Design review of the part built by this model. Coordinates are the model's own, in mm. Round coordinates to 2 decimals unless told otherwise and drop trailing zeros. Write each loop counter-clockwise with the first axis right and the second up, starting at its lowest first coordinate (ties: lowest second). Pieces come first, ordered by that corner, then holes. Notation, with made-up numbers: (59.25, 34.25) - (100.25, 34.25) arc R34 ccw to (100.25, 66.25) - close; hole circle Ø11 at (5.25, -29.75). An arc over 180 degrees is marked (long way). Use one line per item in the form item = value.
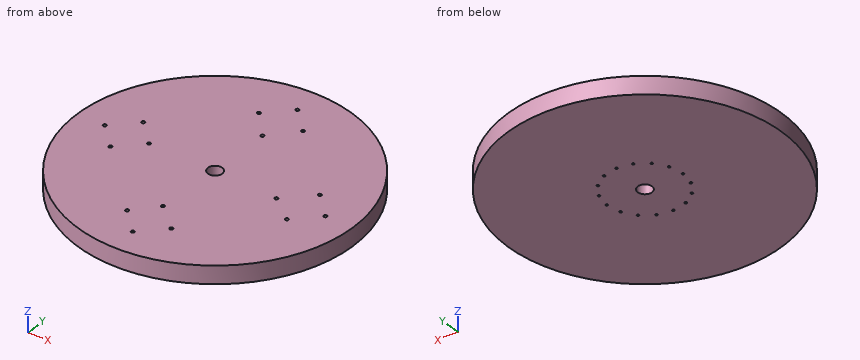
```python
from build123d import *

# Parameters (mm, degrees)
SKETCH_1_R               = 125
EXTRUDE_1_DEPTH          = 8.1
CUT_EXTRUDE_1_DEPTH      = 178.517435763
CUT_EXTRUDE_1_DEPTH_BACK = 178.517435763
SKETCH_3_R               = 6.52
SKETCH_2_R               = 1.03
CUT_EXTRUDE_4_DEPTH      = 10
SKETCH_7_R               = 1.5
CUT_EXTRUDE_5_DEPTH      = 10


with BuildPart() as part:
    # 草图1 → 凸台-拉伸1 (new, symmetric)
    with BuildSketch(Plane.XY):
        Circle(SKETCH_1_R)
    extrude(amount=EXTRUDE_1_DEPTH, both=True)

    # 草图3 → 切除-拉伸1 (cut, two sides: drawn at the far end of the back side and taken through both)
    with BuildSketch(Plane.XY.offset(8.1).offset(-CUT_EXTRUDE_1_DEPTH_BACK)):
        Circle(SKETCH_3_R)
    extrude(amount=CUT_EXTRUDE_1_DEPTH + CUT_EXTRUDE_1_DEPTH_BACK, mode=Mode.SUBTRACT)

    # 草图2 → 切除-拉伸4 (cut)
    with BuildSketch(Plane(origin=(0, 0, -8.1), x_dir=(-1, 0, 0), z_dir=(0, 0, -1))):
        with Locations((0, 34.5)):
            Circle(SKETCH_2_R)
        with Locations((13.202578417, 31.873843872)):
            Circle(SKETCH_2_R)
        with Locations((24.395183951, 24.395183951)):
            Circle(SKETCH_2_R)
        with Locations((31.873843872, 13.202578417)):
            Circle(SKETCH_2_R)
        with Locations((34.5, 0)):
            Circle(SKETCH_2_R)
        with Locations((31.873843872, -13.202578417)):
            Circle(SKETCH_2_R)
        with Locations((24.395183951, -24.395183951)):
            Circle(SKETCH_2_R)
        with Locations((13.202578417, -31.873843872)):
            Circle(SKETCH_2_R)
        with Locations((0, -34.5)):
            Circle(SKETCH_2_R)
        with Locations((-13.202578417, -31.873843872)):
            Circle(SKETCH_2_R)
        with Locations((-24.395183951, -24.395183951)):
            Circle(SKETCH_2_R)
        with Locations((-31.873843872, -13.202578417)):
            Circle(SKETCH_2_R)
        with Locations((-34.5, 0)):
            Circle(SKETCH_2_R)
        with Locations((-31.873843872, 13.202578417)):
            Circle(SKETCH_2_R)
        with Locations((-24.395183951, 24.395183951)):
            Circle(SKETCH_2_R)
        with Locations((-13.202578417, 31.873843872)):
            Circle(SKETCH_2_R)
    extrude(amount=-CUT_EXTRUDE_4_DEPTH, mode=Mode.SUBTRACT)

    # 草图7 → 切除-拉伸5 (cut)
    with BuildSketch(Plane.XY.offset(8.1)):
        with Locations((-100, 0)):
            Circle(SKETCH_7_R)
        with Locations((-80, 20)):
            Circle(SKETCH_7_R)
        with Locations((-60, 0)):
            Circle(SKETCH_7_R)
        with Locations((-80, -20)):
            Circle(SKETCH_7_R)
        with Locations((0, 57.5)):
            Circle(SKETCH_7_R)
        with Locations((57.5, -2.5)):
            Circle(SKETCH_7_R)
        with Locations((-2.5, -60)):
            Circle(SKETCH_7_R)
        with Locations((-20, 80)):
            Circle(SKETCH_7_R)
        with Locations((80, 20)):
            Circle(SKETCH_7_R)
        with Locations((20, -80)):
            Circle(SKETCH_7_R)
        with Locations((20, 80)):
            Circle(SKETCH_7_R)
        with Locations((0, 100)):
            Circle(SKETCH_7_R)
        with Locations((80, -20)):
            Circle(SKETCH_7_R)
        with Locations((100, 0)):
            Circle(SKETCH_7_R)
        with Locations((-20, -80)):
            Circle(SKETCH_7_R)
        with Locations((0, -100)):
            Circle(SKETCH_7_R)
    extrude(amount=-CUT_EXTRUDE_5_DEPTH, mode=Mode.SUBTRACT)


solid = part.part
```
Q1. We need section A-A on z = 5.5. State how many separate pieces and enclosed holes the cut face has, then the cut area to 3 significant figures.
Calculated:
separate_pieces = 1
enclosed_holes = 17
area = 48,800 mm2
Q2. We need section C-C on x = 39. Write out the cut boundary in (y, z), then the cut area to 3 significant figures.
Calculated:
outline = (-118.76, -8.1) - (118.76, -8.1) - (118.76, 8.1) - (-118.76, 8.1) - close
area = 3,850 mm2
Q3. We need section B-B on y = -66.5. Write out the cut boundary in (x, z).
Calculated:
outline = (-105.84, -8.1) - (105.84, -8.1) - (105.84, 8.1) - (-105.84, 8.1) - close
Q4. To check wall thickness, follow line 1 along Y through (x, z) = (0, -3); line 2 along Y through (x, z) = (-80, 4); line 3 along Y through (x, z) = (20, 1). State the ranges of each line that lie inside material, in increasing order. Write a range as from..to.
Calculated:
line_1 = -125..-35.53, -33.47..-6.52, 6.52..33.47, 35.53..125
line_2 = -96.05..-21.5, -18.5..18.5, 21.5..96.05
line_3 = -123.39..-81.5, -78.5..78.5, 81.5..123.39
Q5. For P1, Ø2.5, axis at x = -20, y = -80, coming from the +Z side; P2, Ø4, axis at y = 88, z = -1.5, coming from the -X side; P3, Ø1.5, axis at x = 77.5, z = -1.5, coming from the +Y side, all flat-tipped, find the tip position at first contact; note any pin that passes through.
Calculated:
P1 = -1.9
P2 = -90.71
P3 = 98.66
